Geometry: see drawing. Coordinates: mm, zero at the bounding-box minimum. Round coordinates to 2 decimals unless told otherwise and drop trailing zeros. Write each loop counter-clockwise with the first axis right and the second up, starting at its lowest first coordinate (ties: lowest second). Pieces come first, ordered by that corner, then holes.
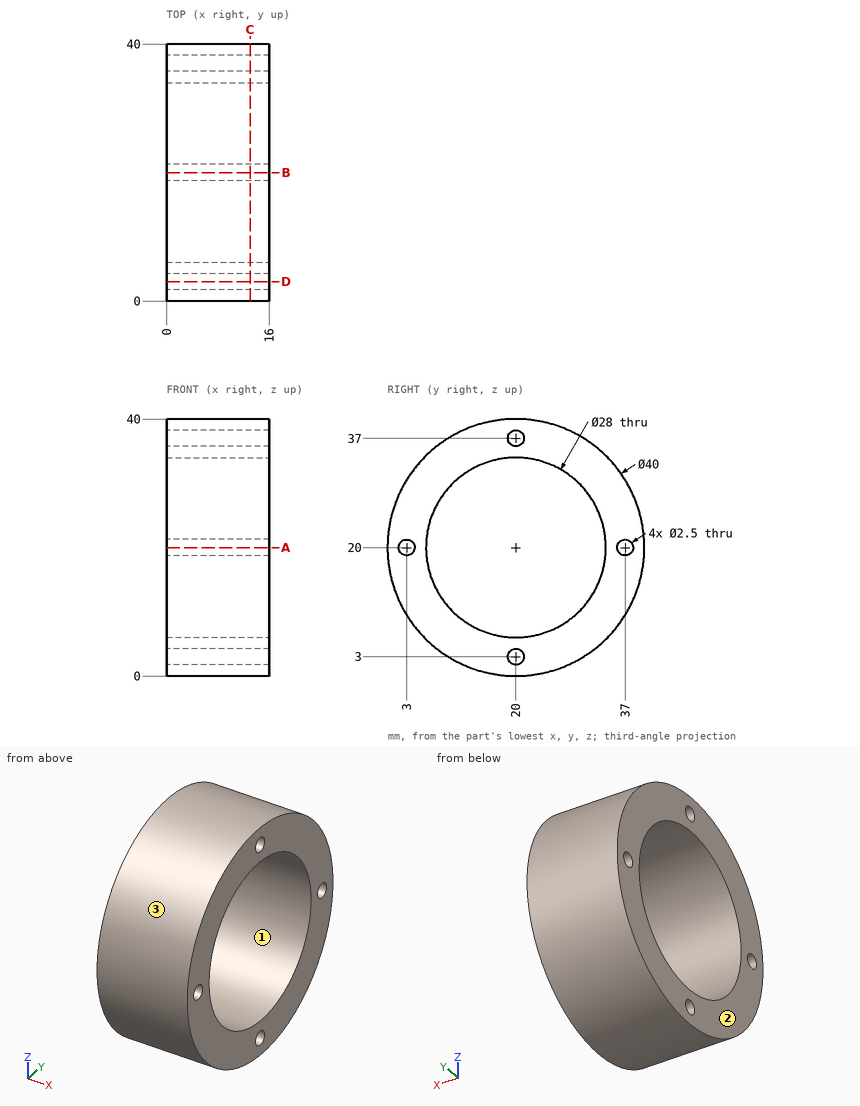
1) Section query C-C on x = 13. Return the cut outline in (y, z).
Taken from the geometry:
outline: circle Ø40 at (20, 20); hole circle Ø2.5 at (3, 20); hole circle Ø28 at (20, 20); hole circle Ø2.5 at (20, 3); hole circle Ø2.5 at (20, 37); hole circle Ø2.5 at (37, 20)
2) Contact query for flat-ended pins moving along their axis: P1, Ø8, axis at x = 9.5, y = 15.5, coming from the -Z side; P2, Ø8, axis at x = 5.5, z = 32, coming from the +Y side; P3, Ø3, axis at x = 3, y = 13, coming from the -Z side; P4, Ø1.5, axis at y = 20, z = 3, coming from the -X side. Output: stop coordinate, or through.
Taken from the geometry:
P1: stops at z = 0.01
P2: stops at y = 38.33
P3: stops at z = 0.77
P4: passes through
3) Section query A-A on z = 20. Return the cut outline in (x, y), then the cut area to 3 significant figures.
Taken from the geometry:
outline: (0, 0) - (16, 0) - (16, 1.75) - (0, 1.75) - close; (0, 4.25) - (16, 4.25) - (16, 6) - (0, 6) - close; (0, 34) - (16, 34) - (16, 35.75) - (0, 35.75) - close; (0, 38.25) - (16, 38.25) - (16, 40) - (0, 40) - close
area: 112 mm2
4) Pull-direction query (Y, two-part tool) for the marked faces 1, 2 and 3; classes: released by +Y, released by -Y, zero draft, split by the parting line, or undercut.
Taken from the geometry:
face 1: undercut
face 2: zero draft
face 3: split by the parting line
5) Section query D-D on y = 3. Return the cut outline in (x, z).
Taken from the geometry:
outline: (0, 9.46) - (16, 9.46) - (16, 18.75) - (0, 18.75) - close; (0, 21.25) - (16, 21.25) - (16, 30.54) - (0, 30.54) - close
6) Material intervals for line 1 (Y direction, x = 4.5, z = 20); line 2 (Z direction, x = 7.75, y = 19); line 3 (Z direction, x = 9, y = 28), sorted ascending.
Taken from the geometry:
line 1: y = 0 to 1.75, 4.25 to 6, 34 to 35.75, 38.25 to 40
line 2: z = 0.03 to 2.25, 3.75 to 6.04, 33.96 to 36.25, 37.75 to 39.97
line 3: z = 1.67 to 8.51, 31.49 to 38.33
